from build123d import *

# Parameters (mm, degrees)
BASE_FLANGE1_DEPTH      = 25.273
CUT_EXTRUDE1_DEPTH      = 117.462097169
CUT_EXTRUDE1_DEPTH_BACK = 117.462097169
SKETCH6_W               = 13.208
SKETCH6_H               = 3.048
CUT_EXTRUDE2_DEPTH      = 182.604935466
CUT_EXTRUDE2_DEPTH_BACK = 182.604935466
SKETCH7_W               = 3.048
SKETCH7_H               = 13.208
FILLET1_R               = 2.54
SKETCH9_R               = 1.5875
SKETCH9_R_2             = 0.7747
CUT_EXTRUDE4_DEPTH      = 182.604935466
CUT_EXTRUDE5_REACH      = 186.328
SKETCH10_R              = 1.651
CUT_EXTRUDE6_REACH      = 186.328
SKETCH11_W              = 3.556
SKETCH11_H              = 13.208
CUT_EXTRUDE8_REACH      = 120.531
SKETCH15_W              = 43.500088515
SKETCH15_H              = 25.146
FILLET2_R               = 5.08
CUT_EXTRUDE9_REACH      = 186.328
CUT_EXTRUDE12_REACH     = 186.328
SKETCH21_W              = 33.274
SKETCH21_H              = 40.343404573
FILLET4_R               = 5.08


# Sheet-metal steps are written as plain solids
with BuildPart() as part:
    # Sketch1 → Base-Flange1 (new, symmetric)
    with BuildSketch(Plane.XY):
        with BuildLine():
            Line((79.441088515, 78.232), (79.441088515, 2.667))
            ThreePointArc((79.441088515, 2.667), (78.6599423, 0.781146215), (76.774088515, 0))
            Line((76.774088515, 0), (-76.774088515, 0))
            ThreePointArc((-76.774088515, 0), (-78.6599423, 0.781146215), (-79.441088515, 2.667))
            Line((-79.441088515, 2.667), (-79.441088515, 78.232))
            Line((-79.441088515, 78.232), (-82.489088515, 78.232))
            Line((-82.489088515, 78.232), (-82.489088515, 2.667))
            ThreePointArc((-82.489088515, 2.667), (-80.815203769, -1.374115254), (-76.774088515, -3.048))
            Line((-76.774088515, -3.048), (76.774088515, -3.048))
            ThreePointArc((76.774088515, -3.048), (80.815203769, -1.374115254), (82.489088515, 2.667))
            Line((82.489088515, 2.667), (82.489088515, 78.232))
            Line((82.489088515, 78.232), (79.441088515, 78.232))
        make_face()
    extrude(amount=BASE_FLANGE1_DEPTH, both=True)

    # Sketch6 → Cut-Extrude1 (cut, two sides: drawn at the far end of the back side and taken through both)
    with BuildSketch(Plane(origin=(0, 0, 0), x_dir=(1, 0, 0), z_dir=(0, 1, 0)).offset(-CUT_EXTRUDE1_DEPTH_BACK)):
        with Locations((-57.404, 23.749)):
            Rectangle(SKETCH6_W, SKETCH6_H)
        with Locations((-57.404, -23.749)):
            Rectangle(SKETCH6_W, SKETCH6_H)
        with Locations((57.404, -23.749)):
            Rectangle(SKETCH6_W, SKETCH6_H)
        with Locations((57.404, 23.749)):
            Rectangle(SKETCH6_W, SKETCH6_H)
    extrude(amount=CUT_EXTRUDE1_DEPTH + CUT_EXTRUDE1_DEPTH_BACK, mode=Mode.SUBTRACT)

    # Sketch7 → Cut-Extrude2 (cut, two sides: drawn at the far end of the back side and taken through both)
    with BuildSketch(Plane(origin=(-79.441088515, 0, 0), x_dir=(0, 0, -1), z_dir=(1, 0, 0)).offset(-CUT_EXTRUDE2_DEPTH_BACK)):
        with Locations((-23.749, 12.446)):
            Rectangle(SKETCH7_W, SKETCH7_H)
        with Locations((23.749, 12.446)):
            Rectangle(SKETCH7_W, SKETCH7_H)
        with Locations((23.749, 64.008)):
            Rectangle(SKETCH7_W, SKETCH7_H)
        with Locations((-23.749, 64.008)):
            Rectangle(SKETCH7_W, SKETCH7_H)
    extrude(amount=CUT_EXTRUDE2_DEPTH + CUT_EXTRUDE2_DEPTH_BACK, mode=Mode.SUBTRACT)

    # Fillet1
    fillet1_edges = [part.edges().sort_by_distance(p)[0] for p in [
        (80.965088515, 78.232, -25.273),
        (-80.965088515, 78.232, -25.273),
        (80.965088515, 78.232, 25.273),
        (-80.965088515, 78.232, 25.273),
    ]]
    fillet(fillet1_edges, radius=FILLET1_R)

    # Sketch9 → Cut-Extrude4 (cut, through all)
    with BuildSketch(Plane.ZY.offset(-79.441088515)):
        with Locations(Location((0, 69.638595427, 0), (0, 0, 270))):
            Circle(SKETCH9_R)
        with Locations(Location((0, 60.113595427, 0), (0, 0, 270))):
            Circle(SKETCH9_R_2)
    extrude(amount=-CUT_EXTRUDE4_DEPTH, mode=Mode.SUBTRACT)

    # Sketch10 → Cut-Extrude5 (cut, up to next)
    with BuildSketch(Plane.ZY.offset(82.489088515), mode=Mode.PRIVATE) as cut_extrude5_sk1:
        with Locations(Location((11.90625, 68.072, 0), (0, 0, 270))):
            Circle(SKETCH10_R)
    cut_extrude5_tool1 = extrude(cut_extrude5_sk1.sketch, amount=-CUT_EXTRUDE5_REACH, mode=Mode.PRIVATE) & part.part
    # Sketch10 → Cut-Extrude5 (cut, up to next)
    with BuildSketch(Plane.ZY.offset(82.489088515), mode=Mode.PRIVATE) as cut_extrude5_sk2:
        with Locations(Location((-11.90625, 68.072, 0), (0, 0, 270))):
            Circle(SKETCH10_R)
    cut_extrude5_tool2 = extrude(cut_extrude5_sk2.sketch, amount=-CUT_EXTRUDE5_REACH, mode=Mode.PRIVATE) & part.part
    add(cut_extrude5_tool1.solids().sort_by_distance((-82.489089, 68.072, 11.90625))[0], mode=Mode.SUBTRACT)
    add(cut_extrude5_tool2.solids().sort_by_distance((-82.489089, 68.072, -11.90625))[0], mode=Mode.SUBTRACT)

    # Sketch11 → Cut-Extrude6 (cut, up to next)
    with BuildSketch(Plane.ZY.offset(82.489088515), mode=Mode.PRIVATE) as cut_extrude6_sk1:
        with Locations((0, 40.132)):
            Rectangle(SKETCH11_W, SKETCH11_H)
    cut_extrude6_tool1 = extrude(cut_extrude6_sk1.sketch, amount=-CUT_EXTRUDE6_REACH, mode=Mode.PRIVATE) & part.part
    add(cut_extrude6_tool1.solids().sort_by_distance((-82.489089, 40.132, 0))[0], mode=Mode.SUBTRACT)

    # Sketch15 → Cut-Extrude8 (cut, up to next)
    with BuildSketch(Plane.XZ.offset(3.048), mode=Mode.PRIVATE) as cut_extrude8_sk1:
        with Locations((-47.404044257, 0)):
            Rectangle(SKETCH15_W, SKETCH15_H)
    cut_extrude8_tool1 = extrude(cut_extrude8_sk1.sketch, amount=-CUT_EXTRUDE8_REACH, mode=Mode.PRIVATE) & part.part
    # Sketch15 → Cut-Extrude8 (cut, up to next)
    with BuildSketch(Plane.XZ.offset(3.048), mode=Mode.PRIVATE) as cut_extrude8_sk2:
        with Locations((47.404044257, 0)):
            Rectangle(SKETCH15_W, SKETCH15_H)
    cut_extrude8_tool2 = extrude(cut_extrude8_sk2.sketch, amount=-CUT_EXTRUDE8_REACH, mode=Mode.PRIVATE) & part.part
    # Sketch15 → Cut-Extrude8 (cut, up to next)
    with BuildSketch(Plane.XZ.offset(3.048), mode=Mode.PRIVATE) as cut_extrude8_sk3:
        with BuildLine():
            Line((12.954, -11.43), (12.954, 11.43))
            ThreePointArc((12.954, 11.43), (12.507630735, 12.507630735), (11.43, 12.954))
            Line((11.43, 12.954), (-11.43, 12.954))
            ThreePointArc((-11.43, 12.954), (-12.507630735, 12.507630735), (-12.954, 11.43))
            Line((-12.954, 11.43), (-12.954, -11.43))
            ThreePointArc((-12.954, -11.43), (-12.507630735, -12.507630735), (-11.43, -12.954))
            Line((-11.43, -12.954), (11.43, -12.954))
            ThreePointArc((11.43, -12.954), (12.507630735, -12.507630735), (12.954, -11.43))
        make_face()
    cut_extrude8_tool3 = extrude(cut_extrude8_sk3.sketch, amount=-CUT_EXTRUDE8_REACH, mode=Mode.PRIVATE) & part.part
    add(cut_extrude8_tool1.solids().sort_by_distance((-47.404044, -3.048, 0))[0], mode=Mode.SUBTRACT)
    add(cut_extrude8_tool2.solids().sort_by_distance((47.404044, -3.048, 0))[0], mode=Mode.SUBTRACT)
    add(cut_extrude8_tool3.solids().sort_by_distance((0, -3.048, 0))[0], mode=Mode.SUBTRACT)

    # Fillet2
    fillet2_edges = [part.edges().sort_by_distance(p)[0] for p in [
        (-69.154088515, -1.524, -12.573),
        (-69.154088515, -1.524, 12.573),
        (-25.654, -1.524, 12.573),
        (-25.654, -1.524, -12.573),
        (25.654, -1.524, 12.573),
        (69.154088515, -1.524, 12.573),
        (69.154088515, -1.524, -12.573),
        (25.654, -1.524, -12.573),
    ]]
    fillet(fillet2_edges, radius=FILLET2_R)

    # Sketch17 → Cut-Extrude9 (cut, up to next)
    with BuildSketch(Plane.ZY.offset(82.489088515), mode=Mode.PRIVATE) as cut_extrude9_sk1:
        with BuildLine():
            Line((-7.1755, 55.372), (-7.1755, 12.827))
            ThreePointArc((-7.1755, 12.827), (-11.90625, 8.09625), (-16.637, 12.827))
            Line((-16.637, 12.827), (-16.637, 55.372))
            ThreePointArc((-16.637, 55.372), (-11.90625, 60.10275), (-7.1755, 55.372))
        make_face()
    cut_extrude9_tool1 = extrude(cut_extrude9_sk1.sketch, amount=-CUT_EXTRUDE9_REACH, mode=Mode.PRIVATE) & part.part
    # Sketch17 → Cut-Extrude9 (cut, up to next)
    with BuildSketch(Plane.ZY.offset(82.489088515), mode=Mode.PRIVATE) as cut_extrude9_sk2:
        with BuildLine():
            Line((7.1755, 55.372), (7.1755, 12.827))
            ThreePointArc((7.1755, 12.827), (11.90625, 8.09625), (16.637, 12.827))
            Line((16.637, 12.827), (16.637, 55.372))
            ThreePointArc((16.637, 55.372), (11.90625, 60.10275), (7.1755, 55.372))
        make_face()
    cut_extrude9_tool2 = extrude(cut_extrude9_sk2.sketch, amount=-CUT_EXTRUDE9_REACH, mode=Mode.PRIVATE) & part.part
    add(cut_extrude9_tool1.solids().sort_by_distance((-82.489089, 34.0995, -11.90625))[0], mode=Mode.SUBTRACT)
    add(cut_extrude9_tool2.solids().sort_by_distance((-82.489089, 34.0995, 11.90625))[0], mode=Mode.SUBTRACT)

    # Sketch21 → Cut-Extrude12 (cut, up to next)
    with BuildSketch(Plane(origin=(82.489088515, 0, 0), x_dir=(0, 0, -1), z_dir=(1, 0, 0)), mode=Mode.PRIVATE) as cut_extrude12_sk1:
        with Locations((0, 30.458702286)):
            Rectangle(SKETCH21_W, SKETCH21_H)
    cut_extrude12_tool1 = extrude(cut_extrude12_sk1.sketch, amount=-CUT_EXTRUDE12_REACH, mode=Mode.PRIVATE) & part.part
    add(cut_extrude12_tool1.solids().sort_by_distance((82.489089, 30.458702, 0))[0], mode=Mode.SUBTRACT)

    # Fillet4
    fillet4_edges = [part.edges().sort_by_distance(p)[0] for p in [
        (80.965088515, 50.630404573, -16.637),
        (80.965088515, 10.287, -16.637),
        (80.965088515, 10.287, 16.637),
        (80.965088515, 50.630404573, 16.637),
    ]]
    fillet(fillet4_edges, radius=FILLET4_R)


solid = part.part
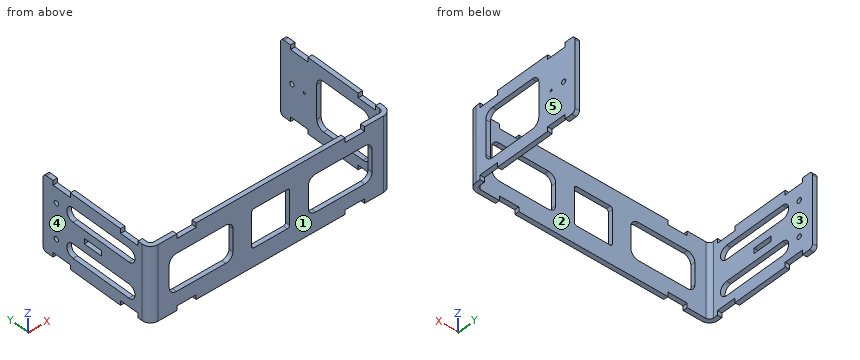
Geometry check sheet. Reference: the model listing, model coordinates, mm. Face numbers are marked on the shaded views. A direction names the side the tool comes from. Coordinates: 2 decimals unless noted, no trailing zeros. Order: outer loops, then holes, each group sorted by start corner. A loop starts at its lowest first (then second) coordinate and runs counter-clockwise, first axis right, second up. Notation, with made-up numbers: (20.5, 31.5) - (52.5, 31.5) arc R21 cw to (52.5, 39.5) - close; hole circle Ø9 at (64, 54). An arc over 180 degrees is marked (long way). One line per item, written item: value.
(1) Thickness scan on probe 1 along X at (y, z) = (64, 12); probe 2 along Y at (x, z) = (-48.5, -19); probe 3 along X at (y, z) = (1, -14.5). Record the ranges inside material, lowest first. Write a range as from..to.
Data:
probe 1: x = -82.49..-79.44, 79.44..82.49
probe 2: y = -3.05..0
probe 3: x = -82.24..-78.86, 78.86..82.24
(2) Sectioned sample at B-B (x = 5). Enter the section's corners in (y, z).
Data:
outline: (-3.05, -25.27) - (0, -25.27) - (0, -12.95) - (-3.05, -12.95) - close; (-3.05, 12.95) - (0, 12.95) - (0, 25.27) - (-3.05, 25.27) - close
(3) Depth check by flat-ended pin: pin 1 Ø3.5 at (x, y) = (-56.5, -1) entering from +Z (3 decimals); pin 2 Ø3.5 at (y, z) = (-2, -3.5) entering from -X; pin 3 Ø0.9 at (y, z) = (-1, 2.5) entering from -X. Enter the tip coordinate at first touch or a pass-through.
Data:
pin 1: stops at z = 22.225
pin 2: stops at x = -81.69
pin 3: stops at x = -81.5
(4) Sectioned sample at C-C (z = -3.5). Enter the section's corners in (x, y) (3 decimals).
Data:
outline: (-82.489, 2.667) arc R5.715 ccw to (-76.774, -3.048) - (-69.154, -3.048) - (-69.154, 0) - (-76.774, 0) arc R2.667 cw to (-79.441, 2.667) - (-79.441, 78.232) - (-82.489, 78.232) - close; (-25.654, -3.048) - (-12.954, -3.048) - (-12.954, 0) - (-25.654, 0) - close; (12.954, -3.048) - (25.654, -3.048) - (25.654, 0) - (12.954, 0) - close; (69.154, -3.048) - (76.774, -3.048) arc R5.715 ccw to (82.489, 2.667) - (82.489, 10.287) - (79.441, 10.287) - (79.441, 2.667) arc R2.667 cw to (76.774, 0) - (69.154, 0) - close; (79.441, 50.63) - (82.489, 50.63) - (82.489, 78.232) - (79.441, 78.232) - close
(5) Sectioned sample at A-A (y = 36). Enter the section's corners in (x, z).
Data:
outline: (-82.49, -25.27) - (-79.44, -25.27) - (-79.44, -16.64) - (-82.49, -16.64) - close; (-82.49, -7.18) - (-79.44, -7.18) - (-79.44, -1.78) - (-82.49, -1.78) - close; (-82.49, 1.78) - (-79.44, 1.78) - (-79.44, 7.18) - (-82.49, 7.18) - close; (-82.49, 16.64) - (-79.44, 16.64) - (-79.44, 25.27) - (-82.49, 25.27) - close; (79.44, -25.27) - (82.49, -25.27) - (82.49, -16.64) - (79.44, -16.64) - close; (79.44, 16.64) - (82.49, 16.64) - (82.49, 25.27) - (79.44, 25.27) - close
(6) Access from +Z, -Z, +X, -X, +Y, -Y to the whole of each face (thin tool, end or side, straight path). Record for the marked faces 1 and 2.
Data:
face 1: +Z, -Z, +X, -X, -Y
face 2: +Z, -Z, +Y
(7) Sectioned sample at D-D (y = 17). Enter the section's corners in (x, z) (1 decimal).
Data:
outline: (-82.5, -22.2) - (-79.4, -22.2) - (-79.4, -16.6) - (-82.5, -16.6) - close; (-82.5, -7.2) - (-79.4, -7.2) - (-79.4, 7.2) - (-82.5, 7.2) - close; (-82.5, 16.6) - (-79.4, 16.6) - (-79.4, 22.2) - (-82.5, 22.2) - close; (79.4, -22.2) - (82.5, -22.2) - (82.5, -16.6) - (79.4, -16.6) - close; (79.4, 16.6) - (82.5, 16.6) - (82.5, 22.2) - (79.4, 22.2) - close
(8) Release check for a two-part mould opening along X. For the marked faces 3, 4 and 5 record: +X half, -X half, draft (parallel to the pull), parting line (faces both ways), or undercut.
Data:
face 3: undercut
face 4: -X half
face 5: +X half
